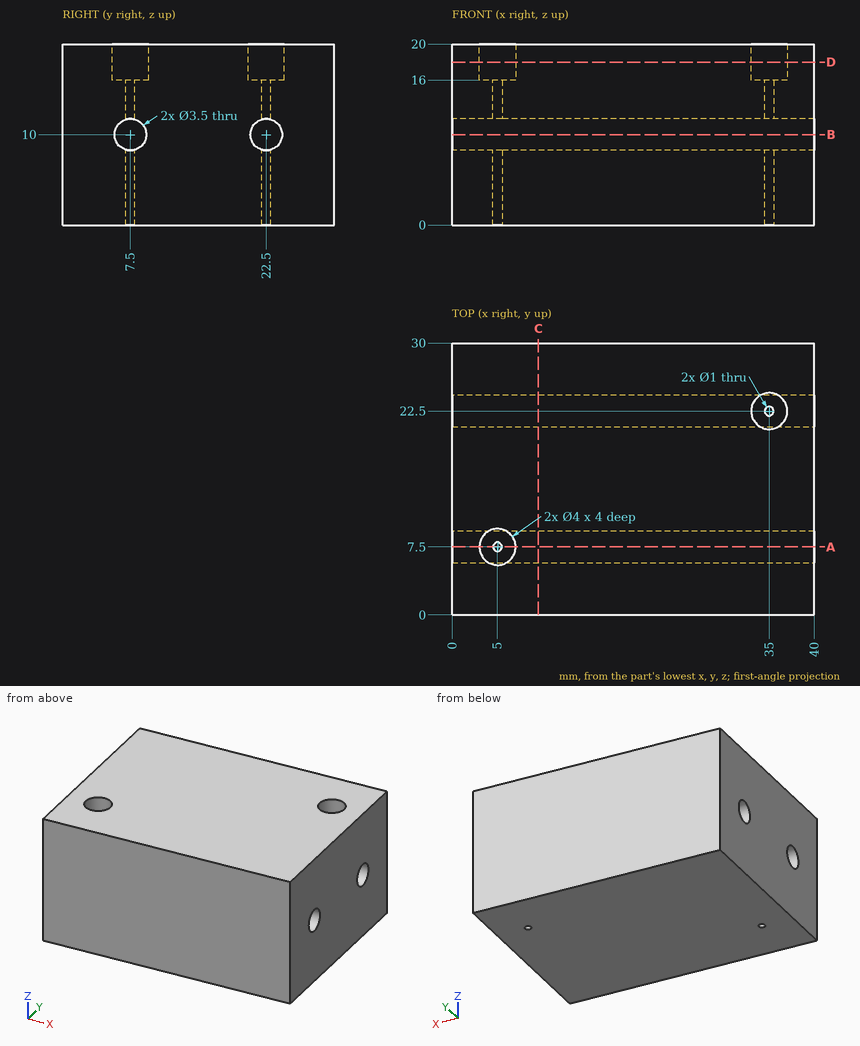
Job drawing, mm, ordinate dimensions from the low corner. One solid piece. Round coordinates to 2 decimals unless told otherwise and drop trailing zeros. Loops run counter-clockwise (first coordinate to the right, second up) from the corner with the lowest first, then second, coordinate; pieces in that order, holes last.
(1) Wall check: line 1 along Y through (x, z) = (35, 14.35); line 2 along Y through (x, z) = (5, 3.5); line 3 along Z through (x, y) = (25, 7.5). Give the ranges that are in metal, low to high.
(2) Cut at A-A (y = 7.5). Give the cut face in (x, z).
(3) Cut at B-B (z = 10). Give the cut face in (x, y), plus the area to 3 significant figures.
(4) Drop flat-ended pins along their axis: pin 1 (8 mm diameter, centred on x = 33, z = 7.5, fed in from -Y); pin 2 (2 mm diameter, centred on y = 22, z = 10.5, fed in from -X). Give the stop position or say it passes through.
(5) Cut at D-D (z = 18). Give the cut face in (x, y), plus the area to 3 significant figures.
(6) Cut at C-C (x = 9.5). Give the cut face in (y, z).
Findings below:
1. line 1: y = 0 to 22, 23 to 30
1. line 2: y = 0 to 7, 8 to 30
1. line 3: z = 0 to 8.25, 11.75 to 20
2. outline: (0, 0) - (4.5, 0) - (4.5, 8.25) - (0, 8.25) - close; (0, 11.75) - (4.5, 11.75) - (4.5, 16) - (3, 16) - (3, 20) - (0, 20) - close; (5.5, 0) - (40, 0) - (40, 8.25) - (5.5, 8.25) - close; (5.5, 11.75) - (40, 11.75) - (40, 20) - (7, 20) - (7, 16) - (5.5, 16) - close
3. outline: (0, 0) - (40, 0) - (40, 5.75) - (0, 5.75) - close; (0, 9.25) - (40, 9.25) - (40, 20.75) - (0, 20.75) - close; (0, 24.25) - (40, 24.25) - (40, 30) - (0, 30) - close
3. area: 920 mm2
4. pin 1: stops at y = 0
4. pin 2: passes through
5. outline: (0, 0) - (40, 0) - (40, 30) - (0, 30) - close; hole circle Ø4 at (5, 7.5); hole circle Ø4 at (35, 22.5)
5. area: 1,170 mm2
6. outline: (0, 0) - (30, 0) - (30, 20) - (0, 20) - close; hole circle Ø3.5 at (7.5, 10); hole circle Ø3.5 at (22.5, 10)
